```python
from build123d import *

# Parameters (mm, degrees)
CROQUIS1_W              = 80
CROQUIS1_H              = 20
CROQUIS1_R              = 2.15
SALIENTE_EXTRUIR1_DEPTH = 20
REDONDEO1_R             = 3


with BuildPart() as part:
    # Croquis1 → Saliente-Extruir1 (new body)
    with BuildSketch(Plane.XY):
        Rectangle(CROQUIS1_W, CROQUIS1_H)
        with Locations((25, 0)):
            Circle(CROQUIS1_R, mode=Mode.SUBTRACT)
        with Locations(Location((-25, 0, 0), (0, 0, 180))):
            Circle(CROQUIS1_R, mode=Mode.SUBTRACT)
    extrude(amount=SALIENTE_EXTRUIR1_DEPTH)

    # Redondeo1
    redondeo1_edges = [part.edges().sort_by_distance(p)[0] for p in [
        (40, 0, 20),
        (0, 10, 20),
        (-40, 0, 20),
        (0, 10, 0),
        (40, 0, 0),
        (0, -10, 0),
        (-40, 0, 0),
        (-40, 10, 10),
        (40, 10, 10),
        (40, -10, 10),
        (-40, -10, 10),
        (0, -10, 20),
    ]]
    fillet(redondeo1_edges, radius=REDONDEO1_R)


solid = part.part
```
The listing builds one solid part. Answer for the finished solid, in the listing's coordinates (mm). Give positions to 0.01 mm unless a question says otherwise; leave off trailing zeros. Order: outer loops, then holes, each group sorted by start corner. A loop starts at its lowest first (then second) coordinate and runs counter-clockwise, first axis right, second up.
1) Find section A-A on y = 0. Write down the section's boundary in (x, z).
Reported:
outline: (-40, 3) arc R3 ccw to (-37, 0) - (-27.15, 0) - (-27.15, 20) - (-37, 20) arc R3 ccw to (-40, 17) - close; (-22.85, 0) - (22.85, 0) - (22.85, 20) - (-22.85, 20) - close; (27.15, 0) - (37, 0) arc R3 ccw to (40, 3) - (40, 17) arc R3 ccw to (37, 20) - (27.15, 20) - close
2) Find section D-D on z = 18.25. Write down the section's boundary in (x, y), then the cut area to 3 significant figures.
Reported:
outline: (-39.73, -7) arc R2.73 ccw to (-37, -9.73) - (37, -9.73) arc R2.73 ccw to (39.73, -7) - (39.73, 7) arc R2.73 ccw to (37, 9.73) - (-37, 9.73) arc R2.73 ccw to (-39.73, 7) - close; hole circle Ø4.3 at (-25, 0); hole circle Ø4.3 at (25, 0)
area: 1,510 mm2
3) Find section C-C on z = 4.5. Write down the section's boundary in (x, y).
Reported:
outline: (-40, -7) arc R3 ccw to (-37, -10) - (37, -10) arc R3 ccw to (40, -7) - (40, 7) arc R3 ccw to (37, 10) - (-37, 10) arc R3 ccw to (-40, 7) - close; hole circle Ø4.3 at (-25, 0); hole circle Ø4.3 at (25, 0)
4) Consider line 1 along X through (y, z) = (0.25, 7.5); line 2 along Y through (x, z) = (-25, 12.5); line 3 along X through (y, z) = (1, 5.75). Determine where each line is inside the solid, lowest interval first.
Reported:
line 1: x = -40 to -27.14, -22.86 to 22.86, 27.14 to 40
line 2: y = -10 to -2.15, 2.15 to 10
line 3: x = -40 to -26.9, -23.1 to 23.1, 26.9 to 40
5) Find section B-B on x = 25. Write down the section's boundary in (y, z).
Reported:
outline: (-10, 3) arc R3 ccw to (-7, 0) - (-2.15, 0) - (-2.15, 20) - (-7, 20) arc R3 ccw to (-10, 17) - close; (2.15, 0) - (7, 0) arc R3 ccw to (10, 3) - (10, 17) arc R3 ccw to (7, 20) - (2.15, 20) - close
6) Determine the mould class of faces 1 (the face through (-39.14, 0.1, 0.9)), 2 (the face through (27.05, 0.65, 9.86)), 3 (the face through (-1, 0, 20)) for opening direction X: pulls with the +X half, pulls with the -X half, needs draft (parallel to the pull), parting line crosses it, or undercut.
Reported:
face 1: pulls with the -X half
face 2: undercut
face 3: needs draft
